Print and shaded views of the part. All mm, measured from the part's lowest x, y and z. A direction names the side the tool comes from. Coordinates: 2 decimals unless noted, no trailing zeros. Loops run counter-clockwise (first coordinate to the right, second up) from the corner with the lowest first, then second, coordinate; pieces in that order, holes last. Notation, with made-up numbers: M 73.5,-12 L 96.5,-12 A10 cw 96.5,7 Z; hole C 47,-39 d5. An arc over 180 degrees is marked long. Use a Markdown table: item, result. Add a question column.
1) Band-saw the part on D-D (y = 7.25). List the corners of the cut face in (x, z), plus the area to 3 significant figures.
2) Tool access for the marked faces 1, 2, 3 and 4: list every direction of +Z, -Z, +X, -X, +Y, -Y with a clear straight run to the whole face (end or side of a thin tool).
3) Wall check: probe 1 along Y at (x, z) = (47, 12); probe 2 along Z at (x, y) = (15, 21.25); probe 3 along Z at (x, y) = (32, 1.5). Give the ranges that are in metal, low to high. Write a range as from..to.
4) Band-saw the part on A-A (y = 13.5). List the corners of the cut face in (x, z), plus the area to 3 significant figures.
5) Pin check, flat tips, straight feed: pin 1 Ø4 at (y, z) = (10, 27) entering from +X; pin 2 Ø2 at (x, y) = (37, 16.5) entering from +Z; pin 3 Ø3 at (x, z) = (48.5, 13.5) entering from -Y. Stop position of each tip, or through.
6) Band-saw the part on B-B (x = 31.75). List the corners of the cut face in (y, z), plus the area to 3 significant figures.
7) Band-saw the part on C-C (z = 14). List the corners of the cut face in (x, y).
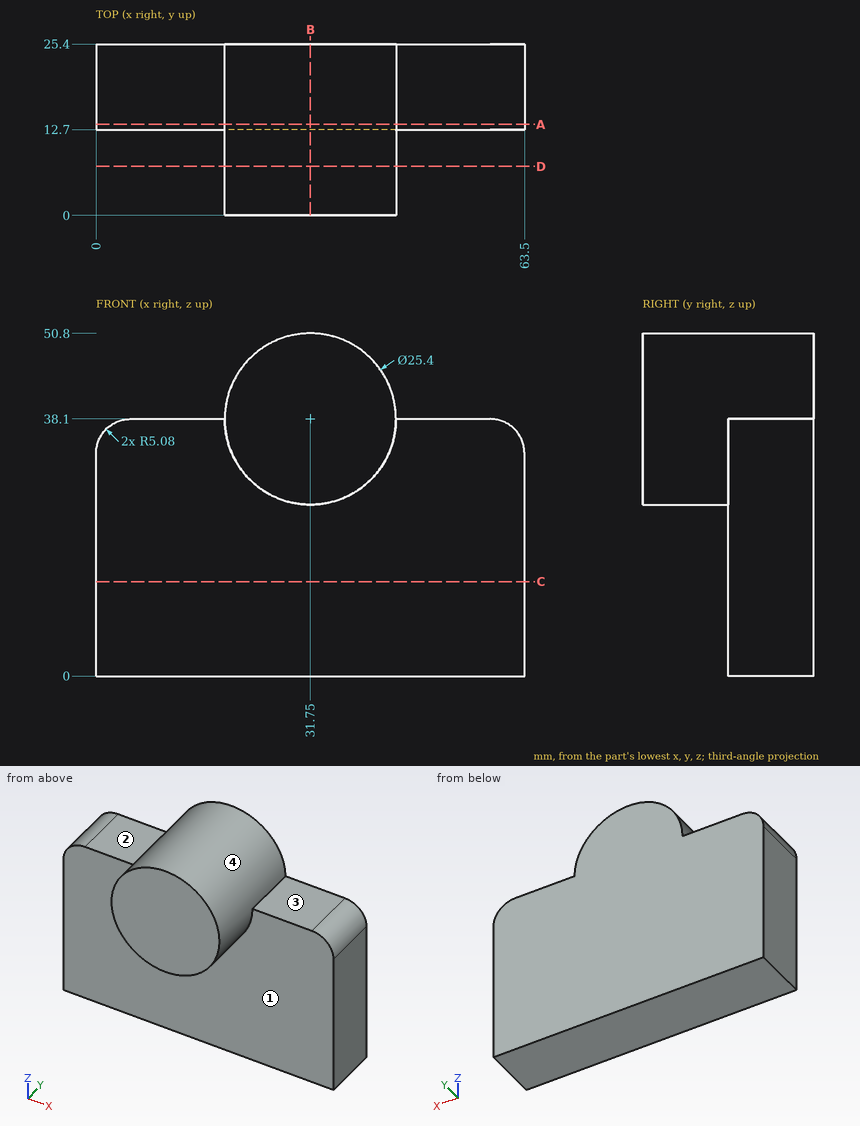
Entries:
| question | item | result |
|---|---|---|
| 1 | outline | C 31.75,38.1 d25.4 |
| 1 | area | 507 mm2 |
| 2 | face 1 | -Z, -Y |
| 2 | face 2 | +Z, -X, +Y, -Y |
| 2 | face 3 | +Z, +X, +Y, -Y |
| 2 | face 4 | -Y |
| 3 | probe 1 | 12.7..25.4 |
| 3 | probe 2 | 0..38.1 |
| 3 | probe 3 | 25.4..50.8 |
| 4 | outline | M 0,0 L 63.5,0 L 63.5,33.02 A5.08 ccw 58.42,38.1 L 44.45,38.1 A12.7 ccw 19.05,38.1 L 5.08,38.1 A5.08 ccw 0,33.02 Z |
| 4 | area | 2,660 mm2 |
| 5 | pin 1 | x = 40.61 |
| 5 | pin 2 | z = 50.07 |
| 5 | pin 3 | y = 12.7 |
| 6 | outline | M 0,25.4 L 12.7,25.4 L 12.7,0 L 25.4,0 L 25.4,50.8 L 0,50.8 Z |
| 6 | area | 968 mm2 |
| 7 | outline | M 0,12.7 L 63.5,12.7 L 63.5,25.4 L 0,25.4 Z |
